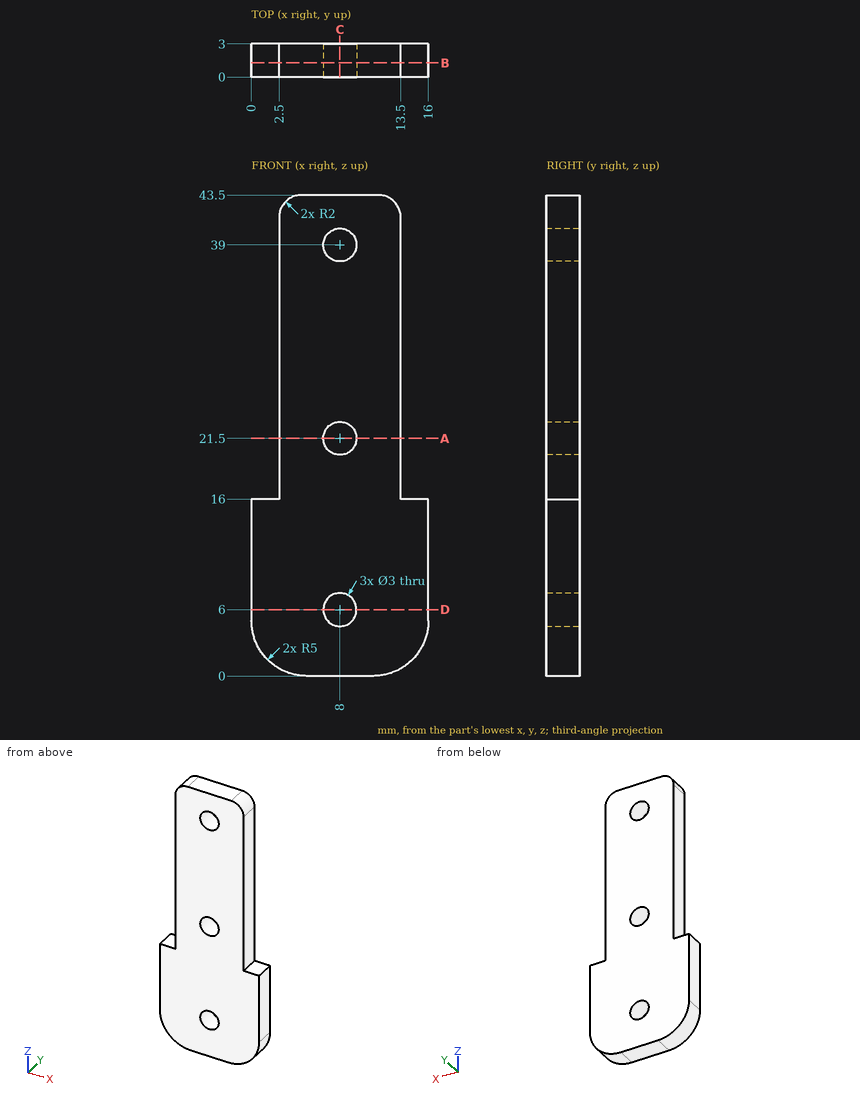
For this review, use the dimensioned drawing (mm, ordinates from the lowest corner) and the shaded views. Give positions to 0.01 mm unless a question says otherwise; leave off trailing zeros. Write each loop counter-clockwise with the first axis right and the second up, starting at its lowest first coordinate (ties: lowest second). Pieces come first, ordered by that corner, then holes. Notation, with made-up numbers: M -27.5,10.25 L 27.5,10.25 A11 ccw 27.5,22.25 Z; hole C 55,59 d8. An arc over 180 degrees is marked long. Answer as a JSON object with one key per item and string values. Group by question number.
1) We need section D-D (z = 6). Give the boundary of the cut face in (x, y), and give its area (3 significant figures).
2) We need section A-A (z = 21.5). Give the boundary of the cut face in (x, y), and give its area (3 significant figures).
3) We need section B-B (y = 1.3). Give the boundary of the cut face in (x, z).
4) We need section C-C (x = 8). Give the boundary of the cut face in (y, z).
5) For line 1 along X through (y, z) = (1.45, 39); line 2 along Z through (x, y) = (7.5, 2.4); line 3 along X through (y, z) = (1.85, 6), list the stretches that pass through material, from the lowest coordinate up.
6) Clearance check with flat-ended pins moving along their axes: pin 1 Ø0.8 at (x, y) = (2, 1.5) entering from +Z; pin 2 Ø1.5 at (y, z) = (2, 26) entering from +X. State where each tip first meets the part, or that it passes through.
Answer key:
{
 "1": {"outline": "M 0,0 L 6.5,0 L 6.5,3 L 0,3 Z; M 9.5,0 L 16,0 L 16,3 L 9.5,3 Z", "area": "39.0 mm²"},
 "2": {"outline": "M 2.5,0 L 6.5,0 L 6.5,3 L 2.5,3 Z; M 9.5,0 L 13.5,0 L 13.5,3 L 9.5,3 Z", "area": "24.0 mm²"},
 "3": {"outline": "M 0,5 A5 ccw 5,0 L 11,0 A5 ccw 16,5 L 16,16 L 13.5,16 L 13.5,41.5 A2 ccw 11.5,43.5 L 4.5,43.5 A2 ccw 2.5,41.5 L 2.5,16 L 0,16 Z; hole C 8,6 d3; hole C 8,21.5 d3; hole C 8,39 d3"},
 "4": {"outline": "M 0,0 L 3,0 L 3,4.5 L 0,4.5 Z; M 0,7.5 L 3,7.5 L 3,20 L 0,20 Z; M 0,23 L 3,23 L 3,37.5 L 0,37.5 Z; M 0,40.5 L 3,40.5 L 3,43.5 L 0,43.5 Z"},
 "5": {"line 1": "x = 2.5 to 6.5, 9.5 to 13.5", "line 2": "z = 0 to 4.59, 7.41 to 20.09, 22.91 to 37.59, 40.41 to 43.5", "line 3": "x = 0 to 6.5, 9.5 to 16"},
 "6": {"pin 1": "stops at z = 16", "pin 2": "stops at x = 13.5"}
}
